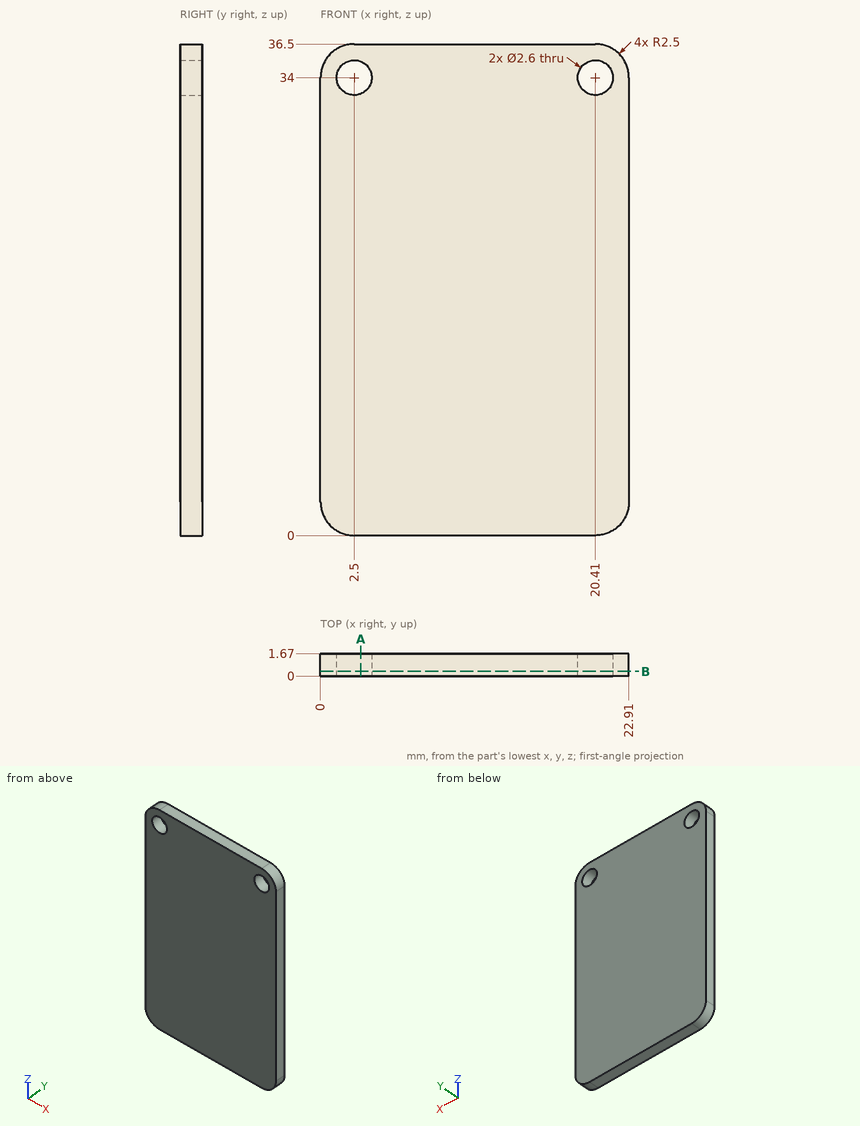
Job drawing, mm, ordinate dimensions from the low corner. One solid piece. Give positions to 0.01 mm unless a question says otherwise; leave off trailing zeros. Order: outer loops, then holes, each group sorted by start corner. A loop starts at its lowest first (then second) coordinate and runs counter-clockwise, first axis right, second up. Notation, with made-up numbers: (-20, 2.5) - (14, 2.5) arc R19 ccw to (14, 8.5) - close; hole circle Ø2 at (20.5, -29). An arc over 180 degrees is marked (long way). One line per question, with ' | ' between items.
1. Drill centre lines: probe 1 along X at (y, z) = (0.4, 34); probe 2 along Z at (x, y) = (2.5, 1.35); probe 3 along Z at (x, y) = (1, 1.2). Where is each one in solid material? Low to high.
Filled in:
probe 1: 0 to 1.2, 3.8 to 19.11, 21.71 to 22.91 | probe 2: 0 to 32.7, 35.3 to 36.5 | probe 3: 0.5 to 36
2. Drop a flat-ended pin along its axis: P1, Ø2, axis at x = 20.41, z = 34, coming from the +Y side (3 decimals). Give the stop position or say it passes through.
Filled in:
P1: through
3. Band-saw the part on B-B on y = 0.35. List the corners of the cut face in (x, z), then the cut area to 3 significant figures.
Filled in:
outline: (0, 2.5) arc R2.5 ccw to (2.5, 0) - (20.41, 0) arc R2.5 ccw to (22.91, 2.5) - (22.91, 34) arc R2.5 ccw to (20.41, 36.5) - (2.5, 36.5) arc R2.5 ccw to (0, 34) - close; hole circle Ø2.6 at (2.5, 34); hole circle Ø2.6 at (20.41, 34) | area: 820 mm²
4. Band-saw the part on A-A on x = 3. List the corners of the cut face in (y, z).
Filled in:
outline: (0, 0) - (1.67, 0) - (1.67, 32.8) - (0, 32.8) - close; (0, 35.2) - (1.67, 35.2) - (1.67, 36.5) - (0, 36.5) - close
